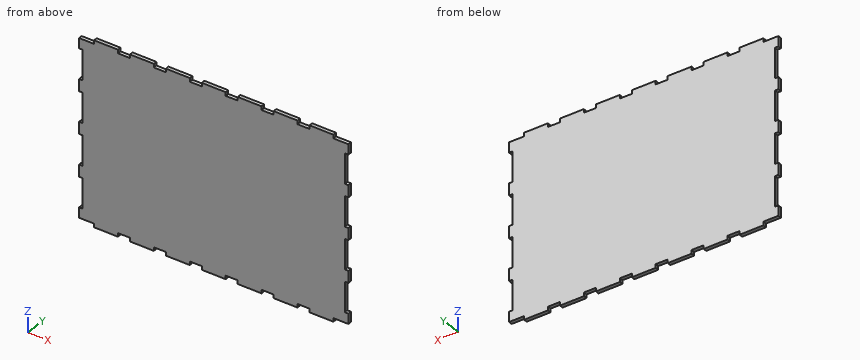
from build123d import *

# Parameters (mm, degrees)
BOSS_EXTRU_1_DEPTH = 6


with BuildPart() as part:
    # Esquisse1 → Boss.-Extru.1 (new body)
    with BuildSketch(Plane(origin=(0, 0, 0), x_dir=(1, 0, 0), z_dir=(0, 1, 0))):
        Polygon((0, 0), (25, 0), (25, -6), (65, -6), (65, 0), (85, 0), (85, -6), (125, -6), (125, 0), (145, 0), (145, -6), (185, -6), (185, 0), (205, 0), (205, -6), (245, -6), (245, 0), (265, 0), (265, -6), (305, -6), (305, 0), (325, 0), (325, -6), (365, -6), (365, 0), (385, 0), (385, -6), (425, -6), (425, 0), (450, 0), (450, 17), (444, 17), (444, 67), (450, 67), (450, 87), (444, 87), (444, 137), (450, 137), (450, 157), (444, 157), (444, 207), (450, 207), (450, 227), (444, 227), (444, 277), (450, 277), (450, 294), (425, 294), (425, 300), (385, 300), (385, 294), (365, 294), (365, 300), (325, 300), (325, 294), (305, 294), (305, 300), (265, 300), (265, 294), (245, 294), (245, 300), (205, 300), (205, 294), (185, 294), (185, 300), (145, 300), (145, 294), (125, 294), (125, 300), (85, 300), (85, 294), (65, 294), (65, 300), (25, 300), (25, 294), (0, 294), (0, 277), (6, 277), (6, 227), (0, 227), (0, 207), (6, 207), (6, 157), (0, 157), (0, 137), (6, 137), (6, 87), (0, 87), (0, 67), (6, 67), (6, 17), (0, 17), align=None)
    extrude(amount=BOSS_EXTRU_1_DEPTH)


solid = part.part
Could you check a few things on this model? Use its own coordinates, in mm. Give positions to 0.01 mm unless a question says otherwise; leave off trailing zeros. Write each loop counter-clockwise with the first axis right and the second up, starting at its lowest first coordinate (ties: lowest second). Pieces come first, ordered by that corner, then holes. Notation, with made-up numbers: (-37.75, -28.75) -> (-18.75, -28.75) arc R32 cw to (-18.75, 10.25) -> close; hole circle Ø5 at (-7.75, 86.5). An arc over 180 degrees is marked (long way). Answer as a JSON object with one key per item and string values.
Q1. Suppose I cut it at A-A on z = -167. Write out the boundary of the cut face in (x, y), then the cut area to 3 significant figures.
Taken from the geometry:
{"outline": "(6, 0) -> (444, 0) -> (444, 6) -> (6, 6) -> close", "area": "2,630 mm²"}
Q2. Will these pins go through, and if not, where does the flat tip stop? pin 1 Ø3 at (x, z) = (212.5, -264) entering from -Y; pin 2 Ø3 at (x, y) = (443, 3.5) entering from +Z; pin 3 Ø3 at (y, z) = (2, 2) entering from -X; pin 4 Ø3 at (x, y) = (447, 4.5) entering from -Z.
Taken from the geometry:
{"pin 1": "stops at y = 0", "pin 2": "stops at z = 0", "pin 3": "stops at x = 25", "pin 4": "stops at z = -294"}
Q3. Please list where these lines run through material, in increasing order: L1, parallel to Z at x = 311.5, y = 0.65; L2, parallel to X at y = 3.55, z = -112.5.
Taken from the geometry:
{"L1": "z = -294 to 0", "L2": "x = 6 to 444"}
